Source: CAD feature listing. Evaluate the final solid. Frame: model axes, mm. A direction names the side the tool comes from. Coordinates: 2 decimals unless noted, no trailing zeros. Loops run counter-clockwise (first coordinate to the right, second up) from the corner with the lowest first, then second, coordinate; pieces in that order, holes last. Notation, with made-up numbers: (-23.5, 44) - (-19.5, 44) arc R20 cw to (-19.5, 53) - close; hole circle Ø8 at (59, -30.75). An arc over 180 degrees is marked (long way). Use CSV: the item, a comma, the result in double quotes. Start each with the question number.
Autodesk Inventor part; units mm, degrees
ref_plane "YZ Plane" through (0, 0, 0) normal (1, 0, 0) x (0, 1, 0)
ref_plane "XZ Plane" through (0, 0, 0) normal (0, 1, 0) x (-1, 0, 0)
ref_plane "XY Plane" through (0, 0, 0) normal (0, 0, 1) x (1, 0, 0)
sketch "Sketch1" plane through (0, 0, 0) normal (0, 0, 1) x (1, 0, 0)
  line L0 (0, 0) -> (80, 0)
  line L1 (80, 0) -> (80, 50)
  line L2 (80, 50) -> (0, 50)
  line L3 (0, 50) -> (0, 0)
  line L4 (12, 40) -> (12, 10) construction
  line L5 (9.25, 40) -> (9.25, 10)
  line L6 (14.75, 10) -> (14.75, 40)
  arc A0 (14.75, 40) -> (9.25, 40) centre (12, 40) ccw
  arc A1 (9.25, 10) -> (14.75, 10) centre (12, 10) ccw
  line L7 (68, 40) -> (68, 10) construction
  line L8 (65.25, 40) -> (65.25, 10)
  line L9 (70.75, 10) -> (70.75, 40)
  arc A2 (70.75, 40) -> (65.25, 40) centre (68, 40) ccw
  arc A3 (65.25, 10) -> (70.75, 10) centre (68, 10) ccw
  point P0 (12, 25)
  point P1 (68, 25)
  dimension "d0" = 80
  dimension "d1" = 50
  dimension "d2" = 5.5
  dimension "d3" = 12
  dimension "d5" = 30
  dimension "d6" = 12
  dimension "d8" = 5.5
  dimension "d9" = 30
  dimension "d38" = 25
  dimension "d39" = 25
extrude "Extrusion1" add sketch "Sketch1" against normal blind 6
sketch "Sketch2" plane through (0, 0, 0) normal (0, 0, 1) x (1, 0, 0)
  line L0 (0, 0) -> (80, 0)
  line L1 (0, 50) -> (0, 0)
  line L2 (0, 50) -> (80, 50)
  point P0 (30, 9.8)
  point P1 (29, 39.8)
  point P2 (51, 39.8)
  point P3 (50, 9.8)
  dimension "d46" = 29
  dimension "d47" = 22
  dimension "d48" = 30
  dimension "d49" = 20
  dimension "d50" = 30
  dimension "d51" = 30
  dimension "d52" = 10.2
  dimension "d53" = 10.2
hole "Hole1" at (30, 9.8, 0) at (29, 39.8, 0) at (51, 39.8, 0) at (50, 9.8, 0) direction (0, 0, -1) diameter 3.4 end through all counterbore diameter 6 counterbore depth 3.4
sketch "Sketch4" plane through (0, 0, 0) normal (0, 0, 1) x (1, 0, 0)
  line L0 (1, 0) -> (79, 0)
  line L1 (54.5, 0) -> (25.5, 0)
  line L2 (25.5, 0) -> (25.5, 3)
  line L3 (25.5, 3) -> (54.5, 3)
  line L4 (54.5, 3) -> (54.5, 0)
  line L5 (80, 1) -> (80, 49)
  point P0 (0, 0)
  dimension "d54" = 3
  dimension "d55" = 25.5
  dimension "d56" = 29
extrude "Extrusion2" cut sketch "Sketch4" against normal through all
properties part number "MountingAdapter"
(1) Ray query, line 1 (X direction, y = 36.5, z = -1.15); line 2 (X direction, y = 9.8, z = -4.7); line 3 (X direction, y = 39.8, z = -1.35). Return the intervals inside material, ascending. Write a range as [from, to].
(2) Section C-C on x = 68. Output: boundary loops of the cut face in (y, z).
(3) Draft query along Y for faces 1 (the flat face through (41, 50, -3)), 2 (the cylindrical face through (11.94, 7.25, -2.96)), 3 (the flat face through (54.5, 2, -3)). Return one class per face: released by +Y, released by -Y, zero draft, split by the parting line, or undercut.
(4) Section B-B on z = -1.35. Output: boundary loops of the cut face in (x, y).
(5) Pin query (flat end, axial travel): pin 1 Ø1 at (x, y) = (46.5, 35.5) entering from +Z; pin 2 Ø4 at (x, y) = (50, 9.8) entering from +Z; pin 3 Ø2.5 at (x, y) = (30, 9.8) entering from -Z; pin 4 Ø3 at (x, z) = (37.5, -3) entering from -Y. Return the tip coordinate at first contact, or that it passes through.
(6) Section A-A on y = 15.5. Output: boundary loops of the cut face in (x, z), plus the area to 3 significant figures.
(7) Section D-D on x = 11.5. Output: boundary loops of the cut face in (y, z).
(8) Reachability of faces 4 (the flat face through (13, 0, -3)), 5 (the cylindrical face through (68.06, 42.75, -2.96)), 6 (the cylindrical face through (48.97, 42.01, -1.72)), 7 (the flat face through (40, 3, -3)) from +Z, -Z, +X, -X, +Y, -Y: full face, straight path, thin tool, end or side. Return the list, or none.
Solution:
1,line 1,"x = [0, 9.25], [14.75, 65.25], [70.75, 80]"
1,line 2,"x = [0, 9.26], [14.74, 28.3], [31.7, 48.3], [51.7, 65.26], [70.74, 80]"
1,line 3,"x = [0, 9.25], [14.75, 26], [32, 48], [54, 65.25], [70.75, 80]"
2,outline,"(0, -6) - (7.25, -6) - (7.25, 0) - (0, 0) - close; (42.75, -6) - (50, -6) - (50, 0) - (42.75, 0) - close"
3,face 1,"released by +Y"
3,face 2,"undercut"
3,face 3,"zero draft"
4,outline,"(0, 0) - (25.5, 0) - (25.5, 3) - (54.5, 3) - (54.5, 0) - (80, 0) - (80, 50) - (0, 50) - close; hole (9.25, 10) arc R2.75 ccw to (14.75, 10) - (14.75, 40) arc R2.75 ccw to (9.25, 40) - close; hole circle Ø6 at (29, 39.8); hole circle Ø6 at (30, 9.8); hole circle Ø6 at (50, 9.8); hole circle Ø6 at (51, 39.8); hole (65.25, 10) arc R2.75 ccw to (70.75, 10) - (70.75, 40) arc R2.75 ccw to (65.25, 40) - close"
5,pin 1,"stops at z = 0"
5,pin 2,"stops at z = -3.4"
5,pin 3,"passes through"
5,pin 4,"stops at y = 3"
6,outline,"(0, -6) - (9.25, -6) - (9.25, 0) - (0, 0) - close; (14.75, -6) - (65.25, -6) - (65.25, 0) - (14.75, 0) - close; (70.75, -6) - (80, -6) - (80, 0) - (70.75, 0) - close"
6,area,"414 mm²"
7,outline,"(0, -6) - (7.3, -6) - (7.3, 0) - (0, 0) - close; (42.7, -6) - (50, -6) - (50, 0) - (42.7, 0) - close"
8,face 4,"+Z, -Z, +X, -X, -Y"
8,face 5,"+Z, -Z"
8,face 6,"+Z"
8,face 7,"+Z, -Z, -Y"
